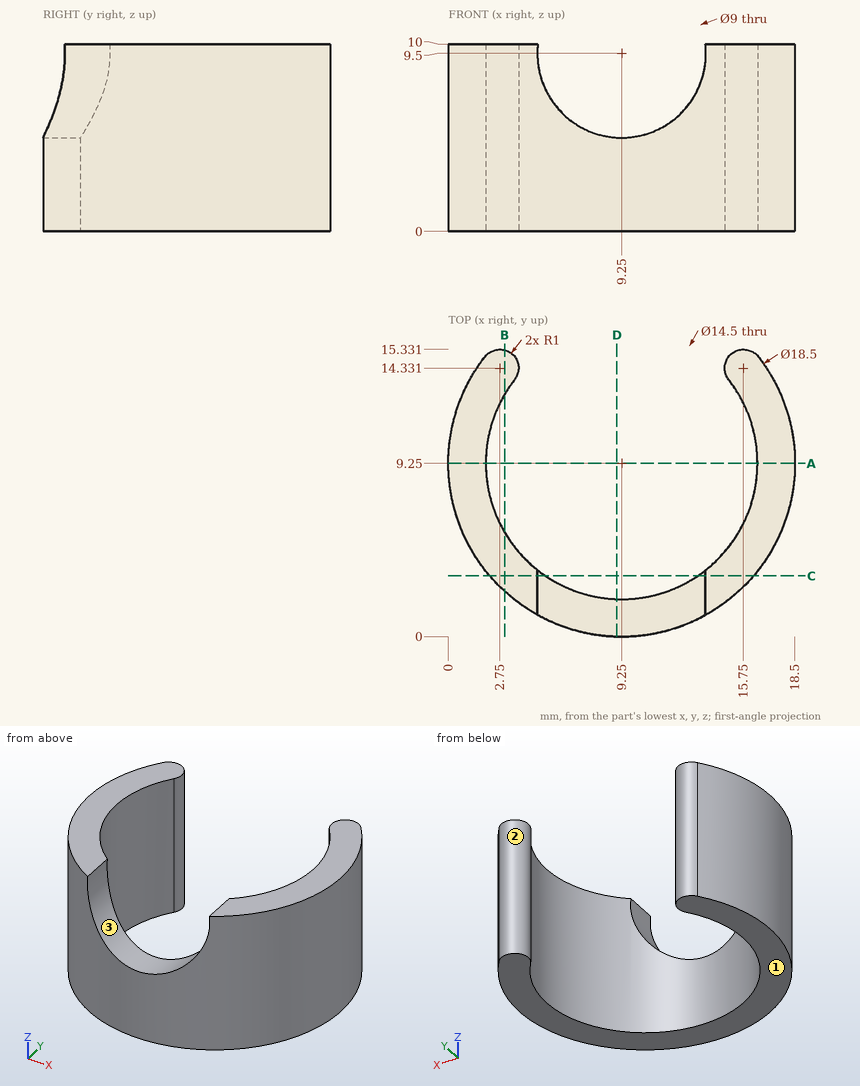
Job drawing, mm, ordinate dimensions from the low corner. One solid piece. Round coordinates to 2 decimals unless told otherwise and drop trailing zeros. Order: outer loops, then holes, each group sorted by start corner. A loop starts at its lowest first (then second) coordinate and runs counter-clockwise, first axis right, second up. Notation, with made-up numbers: M 43,84.25 L 82,84.25 A28 ccw 82,115.25 Z; hole C -24.5,10 d2. An arc over 180 degrees is marked long. Write each question's results on one line, items separated by ' | '. Start each with the question number.
(1) Saw through at D-D, the plane x = 9. Give the cut face in (y, z) (1 decimal).
(2) Drop flat-ended pins along their axis: pin 1 (1.5 mm diameter, centred on x = 8.5, z = 7.5, fed in from -Y); pin 2 (1 mm diameter, centred on x = 12, z = 4, fed in from -Y); pin 3 (1 mm diameter, centred on y = 8.5, z = 8.5, fed in from +X); pin 4 (1.5 mm diameter, centred on y = 3.5, z = 5, fed in from -X). Give the stop position or say it passes through.
(3) Two-plate mould, pull along Z, no slides. Class the marked faces 1, 2 and 3: pulls with the +Z half, pulls with the -Z half, needs draft (parallel to the pull), parting line crosses it, or undercut.
(4) Saw through at C-C, the plane y = 3.25. Give the cut face in (x, z).
(5) Saw through at A-A, the plane y = 9.25. Give the cut face in (x, z).
(6) Probe probe 1 along X at (y, z) = (9.25, 2.25); probe 2 along X at (y, z) = (6.5, 9.5); probe 3 along Y at (x, z) = (3.5, 3.75) (1 decimal). List the from-to ranges inside material, lowest first. Write a range as from..to.
(7) Saw through at B-B, the plane x = 3. Give the cut face in (y, z) (1 decimal), then the cut area to 3 significant figures.
Established:
1) outline: M 0,0 L 2,0 L 2,5 L 0,5 Z
2) pin 1: passes through | pin 2: stops at y = 0.28 | pin 3: stops at x = 18.5 | pin 4: stops at x = 1.47
3) face 1: pulls with the -Z half | face 2: needs draft | face 3: undercut
4) outline: M 2.21,0 L 5.18,0 L 5.18,7.58 A4.5 cw 4.78,10 L 2.21,10 Z; M 13.32,0 L 16.29,0 L 16.29,10 L 13.72,10 A4.5 cw 13.32,7.58 Z
5) outline: M 0,0 L 2,0 L 2,10 L 0,10 Z; M 16.5,0 L 18.5,0 L 18.5,10 L 16.5,10 Z
6) probe 1: x = 0..2, 16.5..18.5 | probe 2: x = 0.42..2.54, 15.96..18.08 | probe 3: y = 2..4.8, 13.7..15
7) outline: M 2.4,0 L 5.6,0 L 5.6,10 L 2.4,10 Z; M 12.9,0 L 15.3,0 L 15.3,10 L 12.9,10 Z | area: 55.2 mm^2
